```python
from build123d import *
from build123d import SkipClean  # not in build123d's __all__

# Parameters (mm, degrees)
F1_DEPTH = 5
F2_R     = 1.5


with BuildPart() as f1:
    # F0 (on Top) → F1 (new body)
    with BuildSketch(Plane.XY):
        with BuildLine():
            ThreePointArc((-2.125, 0), (0, 2.125), (2.125, 0))
            Line((2.125, 0), (29.3, 0))
            Line((29.3, 0), (29.3, 7.41))
            Line((29.3, 7.41), (21.35, 7.41))
            Line((21.35, 7.41), (21.35, 12.66))
            Line((21.35, 12.66), (27.2, 12.66))
            Line((27.2, 12.66), (27.2, 17.36))
            Line((27.2, 17.36), (16.6, 17.36))
            Line((16.6, 17.36), (16.6, 7.41))
            Line((16.6, 7.41), (-24.55, 7.41))
            Line((-24.55, 7.41), (-24.55, 12.66))
            Line((-24.55, 12.66), (-18.7, 12.66))
            Line((-18.7, 12.66), (-18.7, 17.36))
            Line((-18.7, 17.36), (-29.3, 17.36))
            Line((-29.3, 17.36), (-29.3, 0))
            Line((-29.3, 0), (-2.125, 0))
        make_face()
    extrude(amount=F1_DEPTH)

    # F2
    f2_edges = [f1.edges().sort_by_distance(p)[0] for p in [
        (-29.3, 17.36, 2.5),
        (16.6, 17.36, 2.5),
    ]]
    fillet(f2_edges, radius=F2_R)

    # F3: F1 across face


with BuildPart() as f1_1:
    add(f1.part, clean=False)
    with SkipClean():  # cleaning this boolean's faces spoils the solid; the shape is the same uncleaned
        add(f1.part.mirror(Plane(origin=(-15.7125, 0, 2.5), x_dir=(1, 0, 0), z_dir=(0, -1, 0))), clean=False)


solid = f1_1.part
```
Geometry check sheet. Reference: the model listing, model coordinates, mm. A direction names the side the tool comes from. Round coordinates to 2 decimals unless told otherwise and drop trailing zeros. Loops run counter-clockwise (first coordinate to the right, second up) from the corner with the lowest first, then second, coordinate; pieces in that order, holes last. Notation, with made-up numbers: (53.25, 71) - (94.25, 71) arc R13 cw to (94.25, 78) - close; hole circle Ø7 at (11, 31.25). An arc over 180 degrees is marked (long way). Use a Markdown table: item, result.
Q1. Cross-section at A-A on x = -21. Record the cut outline in (y, z).
Solutions:
| item | result |
|---|---|
| outline | (-17.36, 0) - (-12.66, 0) - (-12.66, 5) - (-17.36, 5) - close; (-7.41, 0) - (7.41, 0) - (7.41, 5) - (-7.41, 5) - close; (12.66, 0) - (17.36, 0) - (17.36, 5) - (12.66, 5) - close |
Q2. Cross-section at D-D on x = 0. Record the cut outline in (y, z) (3 decimals).
Solutions:
| item | result |
|---|---|
| outline | (-7.41, 0) - (-2.125, 0) - (-2.125, 5) - (-7.41, 5) - close; (2.125, 0) - (7.41, 0) - (7.41, 5) - (2.125, 5) - close |
Q3. Access from +Z, -Z, +X, -X, +Y, -Y to the whole of each face (thin tool, end or side, straight path). Record for faces 1 (the cylindrical face through (17.05, 16.93, 2.54)), 2 (the flat face through (16.6, -12, 2)), 3 (the flat face through (-24.55, 10, 2)).
Solutions:
| item | result |
|---|---|
| face 1 | +Z, -Z, +Y |
| face 2 | +Z, -Z, -Y |
| face 3 | +Z, -Z |
Q4. Draft check along X on faces 4 (the flat face through (-24.55, -10, 2)), 5 (the flat face through (24, 12.66, 2)), 6 (the flat face through (27.2, 15, 2)). Enter one of: released by +X, released by -X, zero draft, split by the parting line, or undercut.
Solutions:
| item | result |
|---|---|
| face 4 | undercut |
| face 5 | zero draft |
| face 6 | released by +X |
Q5. Go/stop test with flat-tipped pins: P1, Ø2.5, axis at y = 15.5, z = 2, coming from the +X side; P2, Ø3, axis at x = 3, z = 4, coming from the -Y side; P3, Ø2.5, axis at x = -12, z = 2.5, coming from the +Y side. Record where each tip stops, or that it passes through.
Solutions:
| item | result |
|---|---|
| P1 | stops at x = 27.2 |
| P2 | stops at y = -7.41 |
| P3 | stops at y = 7.41 |
Q6. Cross-section at B-B on y = 1.5. Record the cut outline in (x, z).
Solutions:
| item | result |
|---|---|
| outline | (-29.3, 0) - (-1.51, 0) - (-1.51, 5) - (-29.3, 5) - close; (1.51, 0) - (29.3, 0) - (29.3, 5) - (1.51, 5) - close |
Q7. Material ranges on line 1 (Y direction, x = -24, z = 0.4); line 2 (X direction, y = 13.5, z = 4.05); line 3 (X direction, y = 0, z = 2.55) (3 decimals), recorded low to high.
Solutions:
| item | result |
|---|---|
| line 1 | y = -17.36 to -12.66, -7.41 to 7.41, 12.66 to 17.36 |
| line 2 | x = -29.3 to -18.7, 16.6 to 27.2 |
| line 3 | x = -29.3 to -2.125, 2.125 to 29.3 |
